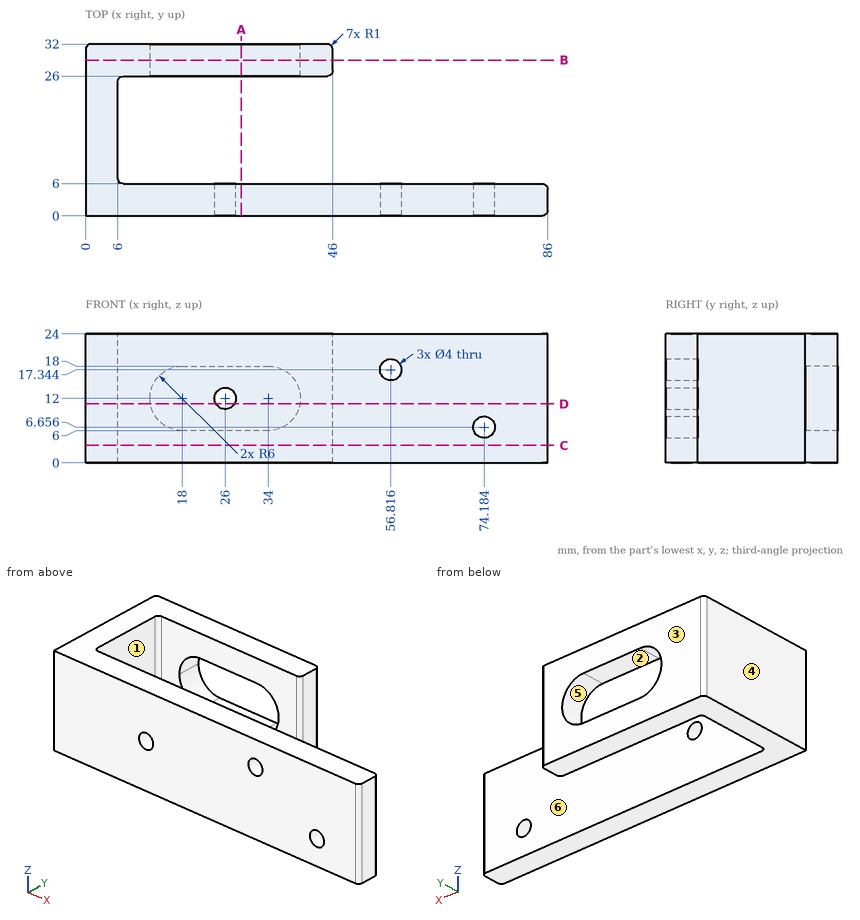
For this review, use the dimensioned drawing (mm, ordinates from the lowest corner) and the shaded views. A direction names the side the tool comes from. Coordinates: 2 decimals unless noted, no trailing zeros. Loops run counter-clockwise (first coordinate to the right, second up) from the corner with the lowest first, then second, coordinate; pieces in that order, holes last. Notation, with made-up numbers: (-22.5, -24) -> (27.5, -24) arc R21 cw to (27.5, 7) -> close; hole circle Ø5 at (43, -13). An arc over 180 degrees is marked (long way). Use a Markdown table: item, result. Add a question column.
1. Add section B-B on y = 29. Write out the cut boundary in (x, z).
2. Add section A-A on x = 29. Write out the cut boundary in (y, z).
3. Add section C-C on z = 3.25. Write out the cut boundary in (x, y).
4. Add section D-D on z = 11. Write out the cut boundary in (x, y).
5. Machinability: for the marked faces 1, 2 and 3, which of the approach directions +Z, -Z, +X, -X, +Y, -Y give a long, thin tool a straight path to every point of the face, cutting with its end or side? Answer none if there is none.
6. To check wall thickness, follow line 1 (Y direction, x = 12.5, z = 18.25); line 2 (Z direction, x = 26, y = 1.5); line 3 (X direction, y = 12, z = 16.25). State the ranges of each line that lie inside material, in increasing order.
7. Draft analysis for pull direction X (two halves, no side actions). For the marked faces 4, 5 and 6, state which applies: pulls with the +X half, pulls with the -X half, needs draft (parallel to the pull), parting line crosses it, or undercut.
8. Clearance check with flat-ended pins moving along their axes: pin 1 Ø1.2 at (y, z) = (29.5, 8) entering from +X; pin 2 Ø1 at (y, z) = (26, 7.5) entering from +X; pin 3 Ø10 at (y, z) = (12.5, 12.5) entering from +X. State where each tip first meets the part, or that it passes through.
Returned:
| question | item | result |
|---|---|---|
| 1 | outline | (0, 0) -> (46, 0) -> (46, 24) -> (0, 24) -> close; hole (18, 6) -> (34, 6) arc R6 ccw to (34, 18) -> (18, 18) arc R6 ccw to start |
| 2 | outline | (0, 0) -> (6, 0) -> (6, 24) -> (0, 24) -> close; (26, 0) -> (32, 0) -> (32, 6) -> (26, 6) -> close; (26, 18) -> (32, 18) -> (32, 24) -> (26, 24) -> close |
| 3 | outline | (0, 0) -> (85, 0) arc R1 ccw to (86, 1) -> (86, 5) arc R1 ccw to (85, 6) -> (7, 6) arc R1 cw to (6, 7) -> (6, 25) arc R1 cw to (7, 26) -> (45, 26) arc R1 ccw to (46, 27) -> (46, 31) arc R1 ccw to (45, 32) -> (1, 32) arc R1 ccw to (0, 31) -> close |
| 4 | outline | (0, 0) -> (24.27, 0) -> (24.27, 6) -> (7, 6) arc R1 cw to (6, 7) -> (6, 25) arc R1 cw to (7, 26) -> (12.08, 26) -> (12.08, 32) -> (1, 32) arc R1 ccw to (0, 31) -> close; (27.73, 0) -> (85, 0) arc R1 ccw to (86, 1) -> (86, 5) arc R1 ccw to (85, 6) -> (27.73, 6) -> close; (39.92, 26) -> (45, 26) arc R1 ccw to (46, 27) -> (46, 31) arc R1 ccw to (45, 32) -> (39.92, 32) -> close |
| 5 | face 1 | +Z, -Z, +X |
| 5 | face 2 | +Y |
| 5 | face 3 | +Z, -Z, +X, -X, +Y |
| 6 | line 1 | y = 0 to 6, 26 to 32 |
| 6 | line 2 | z = 0 to 10, 14 to 24 |
| 6 | line 3 | x = 0 to 6 |
| 7 | face 4 | pulls with the -X half |
| 7 | face 5 | undercut |
| 7 | face 6 | needs draft |
| 8 | pin 1 | stops at x = 46 |
| 8 | pin 2 | stops at x = 45.87 |
| 8 | pin 3 | stops at x = 6 |
